```python
from build123d import *

# Parameters (mm, degrees)
SKETCH2_R          = 15.125
CUT_EXTRUDE5_DEPTH = 24.4
CUT_EXTRUDE6_REACH = 175.705
SKETCH3_R          = 9.543
CUT_EXTRUDE7_REACH = 190.351
SKETCH4_W          = 4.8
SKETCH4_H          = 4.648


with BuildPart() as part:
    # Sketch1 → Revolve1 (revolve)
    with BuildSketch(Plane.XY, mode=Mode.PRIVATE) as revolve1_sk:
        Polygon((-162.990125159, 0), (-162.990125159, 16.125), (-163.990125159, 16.125), (-163.990125159, 37.741454009), (-160.123125159, 37.741454009), (-160.123125159, 102.18499912), (-146.834181255, 102.18499912), (-134.834181255, 30), (-133.834181255, 30), (-121.834181255, 102.18499912), (-105.445019466, 102.18499912), (-105.445019466, 97.18499912), (-87.20655247, 97.18499912), (-87.20655247, 53.18499912), (-47.733023073, 53.18499912), (-42.20655247, 27.18499912), (-42.20655247, 15.17389025), (-43.190125159, 14.993377744), (-43.190125159, 0), align=None)
    revolve(revolve1_sk.sketch.rotate(Axis((-162.990125159, 0, 0), (1, 0, 0)), 90), axis=Axis((-162.990125159, 0, 0), (1, 0, 0)))

    # Sketch2 → Cut-Extrude5 (cut)
    with BuildSketch(Plane.ZY.offset(162.990125159)):
        Circle(SKETCH2_R)
    extrude(amount=-CUT_EXTRUDE5_DEPTH, mode=Mode.SUBTRACT)

    # Sketch3 → Cut-Extrude6 (cut, up to next)
    with BuildSketch(Plane.ZY.offset(138.590125159), mode=Mode.PRIVATE) as cut_extrude6_sk1:
        Circle(SKETCH3_R)
    cut_extrude6_tool1 = extrude(cut_extrude6_sk1.sketch, amount=-CUT_EXTRUDE6_REACH, mode=Mode.PRIVATE) & part.part
    add(cut_extrude6_tool1.solids().sort_by_distance((-138.590125, 0, 0))[0], mode=Mode.SUBTRACT)

    # Sketch4 → Cut-Extrude7 (cut, up to next)
    with BuildSketch(Plane(origin=(-43.190125159, 0, 0), x_dir=(0, 0, -1), z_dir=(1, 0, 0)), mode=Mode.PRIVATE) as cut_extrude7_sk1:
        with Locations((0, -9.543)):
            Rectangle(SKETCH4_W, SKETCH4_H)
    cut_extrude7_tool1 = extrude(cut_extrude7_sk1.sketch, amount=-CUT_EXTRUDE7_REACH, mode=Mode.PRIVATE) & part.part
    add(cut_extrude7_tool1.solids().sort_by_distance((-43.190125, -9.543, 0))[0], mode=Mode.SUBTRACT)


solid = part.part
```
The listing builds one solid part. Answer for the finished solid, in the listing's coordinates (mm). A direction names the side the tool comes from. Round coordinates to 2 decimals unless told otherwise and drop trailing zeros. Loops run counter-clockwise (first coordinate to the right, second up) from the corner with the lowest first, then second, coordinate; pieces in that order, holes last. Notation, with made-up numbers: (60.25, 31) - (67.25, 31) arc R17 cw to (67.25, 48) - close; hole circle Ø8 at (82, 46). An arc over 180 degrees is marked (long way). Use one line per item in the form item = value. Start each with the question number.
1. The part is cut by section A-A on x = -100. Determine the outline of the cut face in (y, z) (3 decimals).
2. Given pin 1 Ø1.3 at (x, y) = (-114.5, -11) entering from -Z; pin 2 Ø1 at (y, z) = (-64.5, 26) entering from -X; pin 3 Ø19.5 at (y, z) = (0, 0) entering from -X, each flat-ended and moving along its own axis, determine where each tip first touches the part or whether it passes through.
3. A tool of negligible diameter and unlimited length cuts with its end or side. For faces 5 (the face through (-42.207, 12, 12)), 6 (the face through (-135.417, -10.064, 31.958)), 7 (the face through (-150.961, -14.765, -3.279)), 8 (the face through (-43.19, 10, 0)), from which of +Z, -Z, +X, -X, +Y, -Y can it reach the whole face along a straight path? Write none if from no direction.
4. Consider line 1 (Y direction, x = -99, z = 0) (3 decimals); line 2 (X direction, y = -76, z = -50); line 3 (X direction, y = 30, z = -57.5). Determine where each line is inside the solid, lowest interval first. Write a range as [from, to].
5. For a pull along Y with two mould halves and no side action, classify faces 1 (the face through (-90, -11.867, 0)), 2 (the face through (-163.5, -4.84, 15.38)), 3 (the face through (-113.525, -30.694, 97.466)), 4 (the face through (-163.99, 16, -8)) as pulls with the +Y half, pulls with the -Y half, needs draft (parallel to the pull), parting line crosses it, or undercut.
Geometry check:
q1.outline = circle Ø194.37 at (0, 0); hole (-11.867, -2.4) - (-9.236, -2.4) arc R9.543 ccw (long way) to (-9.236, 2.4) - (-11.867, 2.4) - close
q2.pin_1 = -101.66
q2.pin_2 = -160.12
q2.pin_3 = -138.59
q3.face_5 = +Z, -Z, +X, +Y, -Y
q3.face_6 = none
q3.face_7 = -X
q3.face_8 = +X
q4.line_1 = [-97.185, -11.867], [9.543, 97.185]
q4.line_2 = [-160.12, -144.97], [-123.7, -87.21]
q4.line_3 = [-160.12, -140.63], [-128.04, -87.21]
q5.face_1 = undercut
q5.face_2 = undercut
q5.face_3 = parting line crosses it
q5.face_4 = needs draft
